Read the model definition and answer for the solid it produces. Units are mm, in the model's axes. Face numbers are marked on the shaded views. Round coordinates to 2 decimals unless told otherwise and drop trailing zeros. Write each loop counter-clockwise with the first axis right and the second up, starting at its lowest first coordinate (ties: lowest second). Pieces come first, ordered by that corner, then holes. Notation, with made-up numbers: (13.5, 79.25) - (61.5, 79.25) arc R36 ccw to (61.5, 116.25) - close; hole circle Ø7 at (57, -33). An arc over 180 degrees is marked (long way). Use one line per item in the form item = value. Start each with the question number.
1) Each of these flat-tipped pins is pushed along its axis until it touches: pin 1 (3 mm diameter, centred on x = 8.5, y = 5, fed in from -Z); pin 2 (3 mm diameter, centred on x = 9, y = 4, fed in from -Z); pin 3 (2 mm diameter, centred on y = 2, z = -7.5, fed in from +X). Where does it stop, or does it pass through?
2) Consider line 1 along Z through (x, y) = (0, 2.5); line 2 along Y through (x, z) = (9, -2.5); line 3 along X through (y, z) = (4, -4.25). Determine where each line is inside the solid, lowest interval first. Write a range as from..to.
3) The part is cut by section C-C, the plane x = 0. Give the vertices of the cut face in (y, z).
4) The part is cut by section D-D, the plane y = 7. Give the vertices of the cut face in (x, z).
5) The part is cut by section A-A, the plane y = 4. Give the vertices of the cut face in (x, z), plus the area to 3 significant figures.
6) The part is cut by section B-B, the plane z = -2.75. Give the vertices of the cut face in (x, y).
7) For a pull along Z with two mould halves and no side action, classify the marked faces 1, 2 and 3 as released by +Z, released by -Z, zero draft, split by the parting line, or undercut.
from build123d import *

# Parameters (mm, degrees)
BOSS_EXTRUDE1_DEPTH         = 8
SKETCH2_R                   = 6
CUT_EXTRUDE1_DEPTH          = 19.761663039
TAP_DRILL_FOR_M3X0_5_TAP1_D = 2.5
SKETCH6_W                   = 12
SKETCH6_H                   = 1
CUT_EXTRUDE2_DEPTH          = 8


with BuildPart() as part:
    # Sketch1 → Boss-Extrude1 (new body)
    with BuildSketch(Plane(origin=(0, 0, 0), x_dir=(1, 0, 0), z_dir=(0, 1, 0))):
        with BuildLine():
            Line((-12, -10), (12, -10))
            Line((12, -10), (12, 0))
            ThreePointArc((12, 0), (0, 12), (-12, 0))
            Line((-12, 0), (-12, -10))
        make_face()
    extrude(amount=BOSS_EXTRUDE1_DEPTH)

    # Sketch2 → Cut-Extrude1 (cut, through all)
    with BuildSketch(Plane(origin=(0, 8, 0), x_dir=(1, 0, 0), z_dir=(0, 1, 0))):
        with Locations(Location((0, 0, 0), (0, 0, 270))):
            Circle(SKETCH2_R)
    extrude(amount=-CUT_EXTRUDE1_DEPTH, mode=Mode.SUBTRACT)

    # Tap Drill for M3x0.5 Tap1 (through all)
    with Locations(Plane.XY.offset(10)):
        with Locations((-9, 4), (9, 4)):
            Hole(TAP_DRILL_FOR_M3X0_5_TAP1_D / 2)

    # Sketch6 → Cut-Extrude2 (cut)
    with BuildSketch(Plane(origin=(0, 8, 0), x_dir=(1, 0, 0), z_dir=(0, 1, 0))):
        with Locations((6, -0.5)):
            Rectangle(SKETCH6_W, SKETCH6_H)
    extrude(amount=-CUT_EXTRUDE2_DEPTH, mode=Mode.SUBTRACT)


solid = part.part
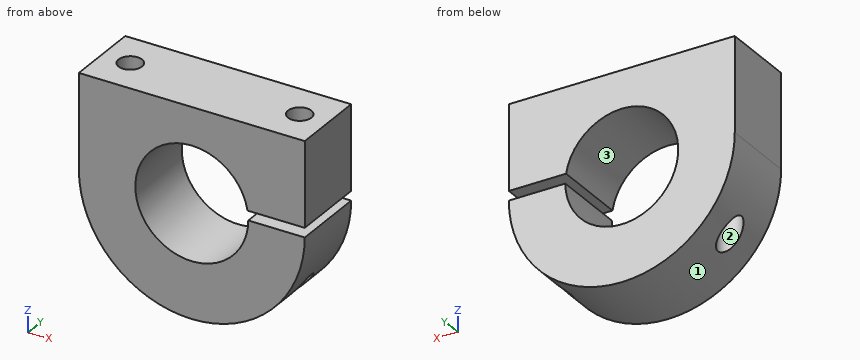
Geometry results:
q1.pin_1 = -9.75
q1.pin_2 = -9.37
q1.pin_3 = 10.09
q2.line_1 = -12..-6, 6..10
q2.line_2 = 0..2.75, 5.25..8
q2.line_3 = -11.22..-10.25, -7.75..-4.24, 4.24..7.75, 10.25..11.22
q3.outline = (0, -12) - (8, -12) - (8, -6) - (0, -6) - close; (0, 6) - (8, 6) - (8, 10) - (0, 10) - close
q4.outline = (-12, 0) arc R12 ccw to (12, 0) - (6, 0) arc R6 cw (long way) to (5.92, 1) - (12, 1) - (12, 10) - (-12, 10) - close
q5.outline = (-12, 0) arc R12 ccw to (-10.25, -6.24) - (-10.25, 10) - (-12, 10) - close; (-7.75, -9.16) arc R12 ccw to (7.75, -9.16) - (7.75, 0) - (6, 0) arc R6 cw (long way) to (5.92, 1) - (7.75, 1) - (7.75, 10) - (-7.75, 10) - close; (10.25, -6.24) arc R12 ccw to (12, 0) - (10.25, 0) - close; (10.25, 1) - (12, 1) - (12, 10) - (10.25, 10) - close
q5.area = 260 mm2
q6.outline = (-11.68, 0) - (-5.33, 0) - (-5.33, 8) - (-11.68, 8) - close; (5.33, 0) - (11.68, 0) - (11.68, 8) - (5.33, 8) - close; hole circle Ø2.5 at (-9, 4); hole circle Ø2.5 at (9, 4)
q7.face_1 = released by -Z
q7.face_2 = zero draft
q7.face_3 = undercut
